The drawing under review shows one solid part. Ordinate dimensions are in mm from its lowest x, y, z. A direction names the side the tool comes from. Round coordinates to 2 decimals unless told otherwise and drop trailing zeros. Write each loop counter-clockwise with the first axis right and the second up, starting at its lowest first coordinate (ties: lowest second). Pieces come first, ordered by that corner, then holes. Notation, with made-up numbers: (88, 77.25) -> (140, 77.25) arc R13 cw to (140, 96.25) -> close; hole circle Ø5 at (17.5, 17). An arc over 180 degrees is marked (long way). Use CSV: the item, a comma, the result in double quotes. Start each with the question number.
1) For pin 1 Ø1 at (y, z) = (2, 1) entering from -X, flat-tipped, find the tip position at first contact; note if it passes through.
2) Wall thickness on probe 1 along X at (y, z) = (3.5, 1.25); probe 2 along Y at (x, z) = (1.5, 1.6): over which ranges is each line inside the solid? List them lowest first. Write a range as [from, to].
3) Machinability: for the marked faces 1, 2 and 3, which of the approach directions +Z, -Z, +X, -X, +Y, -Y give a long, thin tool a straight path to every point of the face, cutting with its end or side? Answer none if there is none.
4) Take a section at A-A, the plane z = 1.45. Give the boundary of the cut face in (x, y), then the cut area to 3 significant figures.
5) Take a section at B-B, the plane y = 5. Give the boundary of the cut face in (x, z).
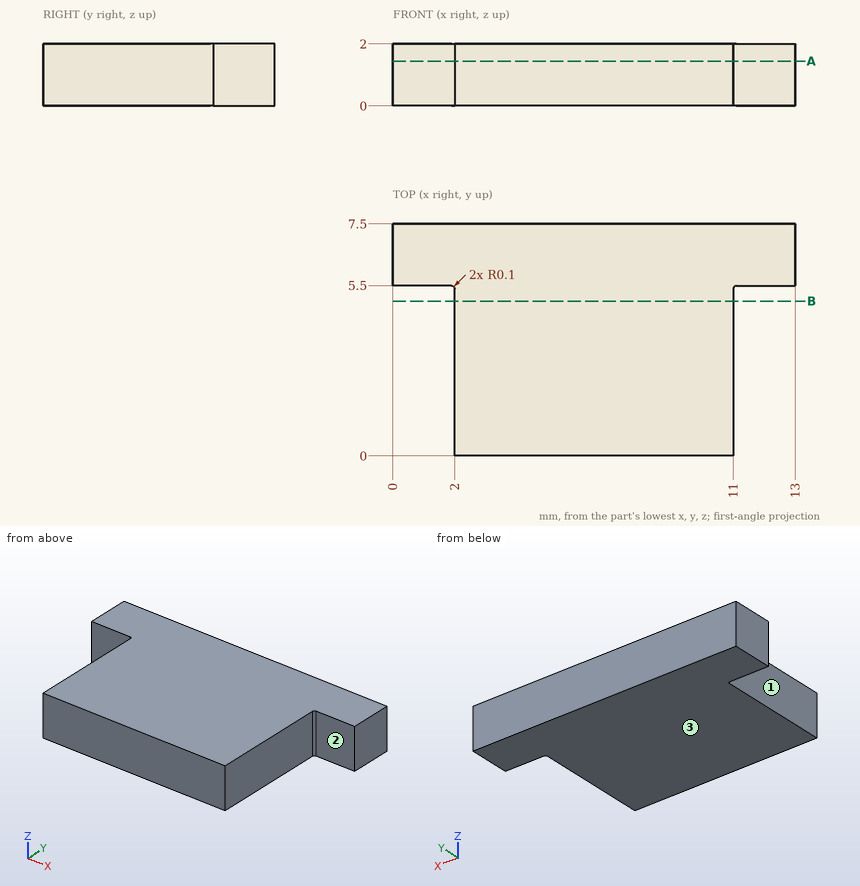
Values found:
1,pin 1,"x = 2"
2,probe 1,"[2, 11]"
2,probe 2,"[5.5, 7.5]"
3,face 1,"+Z, -Z, -X, -Y"
3,face 2,"+Z, -Z, +X, -Y"
3,face 3,"-Z, +X, -X, +Y, -Y"
4,outline,"(0, 5.5) -> (1.9, 5.5) arc R0.1 cw to (2, 5.4) -> (2, 0) -> (11, 0) -> (11, 5.4) arc R0.1 cw to (11.1, 5.5) -> (13, 5.5) -> (13, 7.5) -> (0, 7.5) -> close"
4,area,"75.5 mm²"
5,outline,"(2, 0) -> (11, 0) -> (11, 2) -> (2, 2) -> close"
